from build123d import *

# Parameters (mm, degrees)
SKETCH2_W           = 24
SKETCH2_H           = 24
BOSS_EXTRUDE1_DEPTH = 12
CUT_EXTRUDE1_DEPTH  = 37


with BuildPart() as part:
    # Sketch2 → Boss-Extrude1 (new body)
    with BuildSketch(Plane.XY):
        with Locations((12, 12)):
            Rectangle(SKETCH2_W, SKETCH2_H)
    extrude(amount=BOSS_EXTRUDE1_DEPTH)

    # Sketch4 → Cut-Revolve1 (revolve, cut)
    with BuildSketch(Plane.XY.offset(12)):
        with BuildLine():
            Line((12, 22), (12, 2))
            ThreePointArc((12, 2), (2, 12), (12, 22))
        make_face()
    revolve(axis=Axis((12, 22, 12), (0, -1, 0)), mode=Mode.SUBTRACT)

    # Sketch6 → Cut-Extrude1 (cut, through all)
    with BuildSketch(Plane(origin=(24, 0, 0), x_dir=(0, 0, -1), z_dir=(1, 0, 0))):
        Polygon((0, 24), (-3.026616613, 24), (-5.026616613, 24), (-5.026616613, 0), (-3.026616613, 0), (0, 0), align=None)
    extrude(amount=-CUT_EXTRUDE1_DEPTH, mode=Mode.SUBTRACT)


solid = part.part
Check sheet for the modelled part. Datum: model origin and axes. Units: mm. Round coordinates to 2 decimals unless told otherwise and drop trailing zeros. Order: outer loops, then holes, each group sorted by start corner. A loop starts at its lowest first (then second) coordinate and runs counter-clockwise, first axis right, second up. Notation, with made-up numbers: M -9.5,-13 L 45.5,-13 A22 ccw 45.5,-1 Z; hole C -21,50.25 d6. An arc over 180 degrees is marked long. One line per item, written item: value. Start each with the question number.
1. Scan lines: line 1 along Y through (x, z) = (13.25, 9.5); line 2 along Y through (x, z) = (11.5, 9); line 3 along X through (y, z) = (13.5, 9.25). Record each from-to range of solid material in increasing order.
2. Gauge pin test, flat end, axial feed: P1, Ø10, axis at x = 13, y = 11.5, coming from the -Z side. Record the tip position at first contact, or that the pin passes through.
3. Section check A-A on x = 9. Enter the section's corners in (y, z).
4. Section check B-B on y = 14.5. Enter the section's corners in (x, z), and give its area (3 significant figures).
5. Section check C-C on z = 6. Enter the section's corners in (x, y).
6. Section check D-D on y = 4. Enter the section's corners in (x, z), and give its area (3 significant figures).
Results found:
1. line 1: 0 to 2.4, 21.6 to 24
1. line 2: 0 to 2.47, 21.53 to 24
1. line 3: 0 to 2.5, 21.5 to 24
2. P1: through
3. outline: M 0,5.03 L 5.49,5.03 A9.54 cw 2.46,12 L 0,12 Z; M 18.51,5.03 L 24,5.03 L 24,12 L 21.54,12 A9.54 cw Z
4. outline: M 0,5.03 L 5.28,5.03 A9.68 cw 2.32,12 L 0,12 Z; M 18.72,5.03 L 24,5.03 L 24,12 L 21.68,12 A9.68 cw Z
4. area: 45.1 mm^2
5. outline: M 0,0 L 24,0 L 24,24 L 0,24 Z; hole C 12,12 d16
6. outline: M 0,5.03 L 24,5.03 L 24,12 L 18,12 A6 cw 6,12 L 0,12 Z
6. area: 111 mm^2
